Source: CAD feature listing. Evaluate the final solid. Frame: model axes, mm. Face numbers are marked on the shaded views. A direction names the side the tool comes from. Coordinates: 2 decimals unless noted, no trailing zeros. Loops run counter-clockwise (first coordinate to the right, second up) from the corner with the lowest first, then second, coordinate; pieces in that order, holes last. Notation, with made-up numbers: (-26, 49) - (-19, 49) arc R24 ccw to (-19, 74) - close; hole circle Ø7 at (74, -8.75). An arc over 180 degrees is marked (long way). Use CSV: the item, a comma, the result in double quotes. Start each with the question number.
```python
from build123d import *

# Parameters (mm, degrees)
SKETCH1_W           = 22.5
SKETCH1_H           = 12
BOSS_EXTRUDE1_DEPTH = 11.25
SKETCH3_R           = 6
SKETCH3_R_2         = 2.777492364
BOSS_EXTRUDE3_DEPTH = 4.25
SKETCH4_W           = 4.9
SKETCH4_H           = 12
BOSS_EXTRUDE4_DEPTH = 2.5
SKETCH5_R           = 1.2
CUT_EXTRUDE1_DEPTH  = 2.5
SKETCH6_R           = 0.75
BOSS_EXTRUDE5_DEPTH = 5
SKETCH7_R           = 2.375
BOSS_EXTRUDE6_DEPTH = 3.2
CUT_EXTRUDE2_START  = -3.2
CUT_EXTRUDE2_DEPTH  = 3.2
SKETCH9_R           = 0.925
CUT_EXTRUDE3_DEPTH  = 3.2


with BuildPart() as part:
    # Sketch1 → Boss-Extrude1 (new, symmetric)
    with BuildSketch(Plane(origin=(0, 0, 0), x_dir=(1, 0, 0), z_dir=(0, 1, 0))):
        Rectangle(SKETCH1_W, SKETCH1_H)
    extrude(amount=BOSS_EXTRUDE1_DEPTH, both=True)

    # Sketch3 → Boss-Extrude3 (add)
    with BuildSketch(Plane(origin=(0, 11.25, 0), x_dir=(1, 0, 0), z_dir=(0, 1, 0))):
        with Locations((-5.25, 0)):
            Circle(SKETCH3_R)
        with Locations((0.472507636, 0)):
            Circle(SKETCH3_R_2)
    extrude(amount=BOSS_EXTRUDE3_DEPTH)

    # Sketch4 → Boss-Extrude4 (add)
    with BuildSketch(Plane(origin=(0, 6.95, 0), x_dir=(1, 0, 0), z_dir=(0, 1, 0))):
        with Locations((13.7, 0)):
            Rectangle(SKETCH4_W, SKETCH4_H)
    boss_extrude4 = extrude(amount=-BOSS_EXTRUDE4_DEPTH)

    # Sketch5 → Cut-Extrude1 (cut)
    with BuildSketch(Plane(origin=(0, 6.95, 0), x_dir=(1, 0, 0), z_dir=(0, 1, 0))):
        with BuildLine():
            Line((16.15, -0.75), (16.15, 0.75))
            Line((16.15, 0.75), (14.5867497, 0.75))
            ThreePointArc((14.5867497, 0.75), (14.782276388, 0.397429466), (14.85, 0))
            ThreePointArc((14.85, 0), (14.782276388, -0.397429466), (14.5867497, -0.75))
            Line((14.5867497, -0.75), (16.15, -0.75))
        make_face()
        with Locations((13.65, 0)):
            Circle(SKETCH5_R)
    cut_extrude1 = extrude(amount=-CUT_EXTRUDE1_DEPTH, mode=Mode.SUBTRACT)

    # Mirror1: Boss-Extrude4, Cut-Extrude1 across plane
    add(boss_extrude4.mirror(Plane(origin=(0, 0, 0), x_dir=(0, 0, 1), z_dir=(1, 0, 0))))
    add(cut_extrude1.mirror(Plane(origin=(0, 0, 0), x_dir=(0, 0, 1), z_dir=(1, 0, 0))), mode=Mode.SUBTRACT)

    # Sketch6 → Boss-Extrude5 (add)
    with BuildSketch(Plane.ZY.offset(11.25)):
        with Locations(Location((0, -6.75, 0), (0, 0, 180))):
            Circle(SKETCH6_R)
        with Locations(Location((1.55, -6.75, 0), (0, 0, 180))):
            Circle(SKETCH6_R)
        with Locations(Location((-1.55, -6.75, 0), (0, 0, 180))):
            Circle(SKETCH6_R)
    extrude(amount=BOSS_EXTRUDE5_DEPTH)

    # Sketch7 → Boss-Extrude6 (add)
    with BuildSketch(Plane(origin=(0, 15.5, 0), x_dir=(1, 0, 0), z_dir=(0, 1, 0))):
        with Locations(Location((-5.25, 0, 0), (0, 0, 270))):
            Circle(SKETCH7_R)
    extrude(amount=BOSS_EXTRUDE6_DEPTH)

    # Sketch8 → Cut-Extrude2 (cut)
    with BuildSketch(Plane(origin=(0, 18.7, 0), x_dir=(1, 0, 0), z_dir=(0, 1, 0)).offset(CUT_EXTRUDE2_START)):
        with BuildLine():
            ThreePointArc((-4.939008874, 2.354550811), (-5.25, 2.375), (-5.560991126, 2.354550811))
            Line((-5.560991126, 2.354550811), (-5.25, 2.175))
            Line((-5.25, 2.175), (-4.939008874, 2.354550811))
        make_face()
        with BuildLine():
            ThreePointArc((-4.258809302, 2.158278481), (-4.549956461, 2.269485414), (-4.853158628, 2.341610968))
            Line((-4.853158628, 2.341610968), (-4.608907496, 2.078370853))
            Line((-4.608907496, 2.078370853), (-4.258809302, 2.158278481))
        make_face()
        with BuildLine():
            ThreePointArc((-3.666681374, 1.770233636), (-3.912114862, 1.962317089), (-4.180587228, 2.120608715))
            Line((-4.180587228, 2.120608715), (-4.024778874, 1.797069334))
            Line((-4.024778874, 1.797069334), (-3.666681374, 1.770233636))
        make_face()
        with BuildLine():
            ThreePointArc((-3.215238254, 1.224895765), (-3.393150229, 1.480788279), (-3.603037845, 1.711181072))
            Line((-3.603037845, 1.711181072), (-3.549516526, 1.356090319))
            Line((-3.549516526, 1.356090319), (-3.215238254, 1.224895765))
        make_face()
        with BuildLine():
            ThreePointArc((-2.944592644, 0.570720529), (-3.039174847, 0.867684933), (-3.171828277, 1.149707481))
            Line((-3.171828277, 1.149707481), (-3.225349597, 0.794616728))
            Line((-3.225349597, 0.794616728), (-2.944592644, 0.570720529))
        make_face()
        with BuildLine():
            ThreePointArc((-2.878792595, -0.13416573), (-2.881640982, 0.177483972), (-2.925273387, 0.486077335))
            Line((-2.925273387, 0.486077335), (-3.081081741, 0.162537954))
            Line((-3.081081741, 0.162537954), (-2.878792595, -0.13416573))
        make_face()
        with BuildLine():
            ThreePointArc((-3.02368473, -0.827130775), (-2.934546209, -0.528487218), (-2.885280658, -0.220742916))
            Line((-2.885280658, -0.220742916), (-3.129531791, -0.483983031))
            Line((-3.129531791, -0.483983031), (-3.02368473, -0.827130775))
        make_face()
        with BuildLine():
            ThreePointArc((-3.366394747, -1.446601621), (-3.193189666, -1.1875), (-3.05540362, -0.907949189))
            Line((-3.05540362, -0.907949189), (-3.366394747, -1.0875))
            Line((-3.366394747, -1.0875), (-3.366394747, -1.446601621))
        make_face()
        with BuildLine():
            ThreePointArc((-3.876471356, -1.937535565), (-3.634589748, -1.740998196), (-3.420526102, -1.514480193))
            Line((-3.420526102, -1.514480193), (-3.770624295, -1.594387821))
            Line((-3.770624295, -1.594387821), (-3.876471356, -1.937535565))
        make_face()
        with BuildLine():
            ThreePointArc((-4.508592013, -2.256310971), (-4.21952612, -2.139801061), (-3.948205367, -1.986442985))
            Line((-3.948205367, -1.986442985), (-4.306302867, -1.959607288))
            Line((-4.306302867, -1.959607288), (-4.508592013, -2.256310971))
        make_face()
        with BuildLine():
            ThreePointArc((-5.206590024, -2.374603246), (-4.896024618, -2.348473212), (-4.591554799, -2.281901601))
            Line((-4.591554799, -2.281901601), (-4.925833071, -2.150707047))
            Line((-4.925833071, -2.150707047), (-5.206590024, -2.374603246))
        make_face()
        with BuildLine():
            ThreePointArc((-5.908445201, -2.281901601), (-5.603975382, -2.348473212), (-5.293409976, -2.374603246))
            Line((-5.293409976, -2.374603246), (-5.574166929, -2.150707047))
            Line((-5.574166929, -2.150707047), (-5.908445201, -2.281901601))
        make_face()
        with BuildLine():
            ThreePointArc((-6.551794633, -1.986442985), (-6.28047388, -2.139801061), (-5.991407987, -2.256310971))
            Line((-5.991407987, -2.256310971), (-6.193697133, -1.959607288))
            Line((-6.193697133, -1.959607288), (-6.551794633, -1.986442985))
        make_face()
        with BuildLine():
            ThreePointArc((-7.079473898, -1.514480193), (-6.865410252, -1.740998196), (-6.623528644, -1.937535565))
            Line((-6.623528644, -1.937535565), (-6.729375705, -1.594387821))
            Line((-6.729375705, -1.594387821), (-7.079473898, -1.514480193))
        make_face()
        with BuildLine():
            ThreePointArc((-7.44459638, -0.907949189), (-7.306810334, -1.1875), (-7.133605253, -1.446601621))
            Line((-7.133605253, -1.446601621), (-7.133605253, -1.0875))
            Line((-7.133605253, -1.0875), (-7.44459638, -0.907949189))
        make_face()
        with BuildLine():
            ThreePointArc((-7.614719342, -0.220742916), (-7.565453791, -0.528487218), (-7.47631527, -0.827130775))
            Line((-7.47631527, -0.827130775), (-7.370468209, -0.483983031))
            Line((-7.370468209, -0.483983031), (-7.614719342, -0.220742916))
        make_face()
        with BuildLine():
            ThreePointArc((-7.574726613, 0.486077335), (-7.618359018, 0.177483972), (-7.621207405, -0.13416573))
            Line((-7.621207405, -0.13416573), (-7.418918259, 0.162537954))
            Line((-7.418918259, 0.162537954), (-7.574726613, 0.486077335))
        make_face()
        with BuildLine():
            ThreePointArc((-7.328171723, 1.149707481), (-7.460825153, 0.867684933), (-7.555407356, 0.570720529))
            Line((-7.555407356, 0.570720529), (-7.274650403, 0.794616728))
            Line((-7.274650403, 0.794616728), (-7.328171723, 1.149707481))
        make_face()
        with BuildLine():
            ThreePointArc((-6.896962155, 1.711181072), (-7.106849771, 1.480788279), (-7.284761746, 1.224895765))
            Line((-7.284761746, 1.224895765), (-6.950483474, 1.356090319))
            Line((-6.950483474, 1.356090319), (-6.896962155, 1.711181072))
        make_face()
        with BuildLine():
            ThreePointArc((-6.319412772, 2.120608715), (-6.587885138, 1.962317089), (-6.833318626, 1.770233636))
            Line((-6.833318626, 1.770233636), (-6.475221126, 1.797069334))
            Line((-6.475221126, 1.797069334), (-6.319412772, 2.120608715))
        make_face()
        with BuildLine():
            ThreePointArc((-5.646841372, 2.341610968), (-5.950043539, 2.269485414), (-6.241190698, 2.158278481))
            Line((-6.241190698, 2.158278481), (-5.891092504, 2.078370853))
            Line((-5.891092504, 2.078370853), (-5.646841372, 2.341610968))
        make_face()
    extrude(amount=CUT_EXTRUDE2_DEPTH, mode=Mode.SUBTRACT)

    # Sketch9 → Cut-Extrude3 (cut)
    with BuildSketch(Plane(origin=(0, 18.7, 0), x_dir=(1, 0, 0), z_dir=(0, 1, 0))):
        with Locations(Location((-5.25, 0, 0), (0, 0, 270))):
            Circle(SKETCH9_R)
    extrude(amount=-CUT_EXTRUDE3_DEPTH, mode=Mode.SUBTRACT)


solid = part.part
```
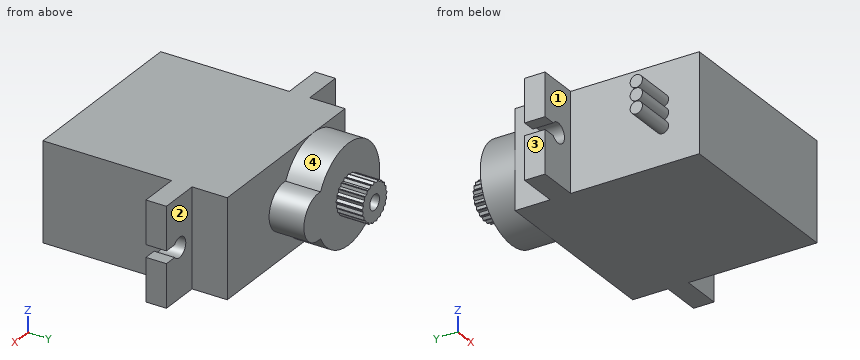
(1) Section C-C on y = -6.75. Output: boundary loops of the cut face in (x, z), plus the area to 4 significant figures.
(2) Reachability of the marked faces 1, 2, 3 and 4 from +Z, -Z, +X, -X, +Y, -Y: full face, straight path, thin tool, end or side. Return the list, or none.
(3) Pin query (flat end, axial travel): pin 1 Ø0.8 at (y, z) = (5, 3.5) entering from -X; pin 2 Ø3 at (x, z) = (-13.65, 0) entering from +Y; pin 3 Ø0.6 at (x, z) = (-5.5, 0) entering from +Y. Return the tip coordinate at first contact, or that it passes through.
(4) Section A-A on x = -13.65. Output: boundary loops of the cut face in (y, z), plus the area to 3 significant figures.
(5) Section B-B on x = 13.65. Output: boundary loops of the cut face in (y, z).
(6) Ray query, line 1 (Z direction, x = 13.65, y = 5.9); line 2 (X direction, y = 5.15, z = 0); line 3 (X direction, y = -7, z = -1.5). Return the intervals inside material, ascending. Write a range as [from, to].
(7) Section D-D on z = 5.5. Output: boundary loops of the cut face in (x, y).
Solution:
1,outline,"(-16.25, -2.3) - (-11.25, -2.3) - (-11.25, -6) - (11.25, -6) - (11.25, 6) - (-11.25, 6) - (-11.25, 2.3) - (-16.25, 2.3) - (-16.25, 0.8) - (-11.25, 0.8) - (-11.25, 0.75) - (-16.25, 0.75) - (-16.25, -0.75) - (-11.25, -0.75) - (-11.25, -0.8) - (-16.25, -0.8) - close"
1,area,"292.5 mm²"
2,face 1,"+Z, -Z, -X"
2,face 2,"+Z, -Z, +X, +Y"
2,face 3,"+Z, -Z, -X, +Y"
2,face 4,"+Y"
3,pin 1,"stops at x = -16.15"
3,pin 2,"stops at y = 6.95"
3,pin 3,"stops at y = 15.5"
4,outline,"circle Ø1.5 at (-6.75, -1.55); circle Ø1.5 at (-6.75, 0); circle Ø1.5 at (-6.75, 1.55); (4.45, -6) - (6.95, -6) - (6.95, -1.2) - (4.45, -1.2) - close; (4.45, 1.2) - (6.95, 1.2) - (6.95, 6) - (4.45, 6) - close"
4,area,"29.3 mm²"
5,outline,"(4.45, -6) - (6.95, -6) - (6.95, -1.2) - (4.45, -1.2) - close; (4.45, 1.2) - (6.95, 1.2) - (6.95, 6) - (4.45, 6) - close"
6,line 1,"z = [-6, -1.2], [1.2, 6]"
6,line 2,"x = [-12.45, 12.45]"
6,line 3,"x = [-16.25, 11.25]"
7,outline,"(-16.15, 4.45) - (-11.25, 4.45) - (-11.25, -11.25) - (11.25, -11.25) - (11.25, 4.45) - (16.15, 4.45) - (16.15, 6.95) - (11.25, 6.95) - (11.25, 11.25) - (-2.85, 11.25) - (-2.85, 15.5) - (-7.65, 15.5) - (-7.65, 11.25) - (-11.25, 11.25) - (-11.25, 6.95) - (-16.15, 6.95) - close"
